Design review of the part built by this model. Coordinates are the model's own, in mm. A direction names the side the tool comes from. Round coordinates to 2 decimals unless told otherwise and drop trailing zeros. Loops run counter-clockwise (first coordinate to the right, second up) from the corner with the lowest first, then second, coordinate; pieces in that order, holes last. Notation, with made-up numbers: (87.5, 30) - (108.5, 30) arc R26 cw to (108.5, 54) - close; hole circle Ø7 at (-4.75, 58). An arc over 180 degrees is marked (long way). Return JSON: item names as keys, results as strings. Group by question number.
Autodesk Inventor part; units mm, degrees
ref_plane "Work Plane1" through (15, 0, 0) normal (0, 0, -1) x (-1, 0, 0)
ref_plane "YZ Plane" through (0, 0, 0) normal (1, 0, 0) x (0, 1, 0)
ref_plane "XZ Plane" through (0, 0, 0) normal (0, 1, 0) x (-1, 0, 0)
sketch "Sketch1" plane through (0, 0, 0) normal (0, 1, 0) x (-1, 0, 0)
  line L0 (-15, -17) -> (15, -17)
  line L1 (15, -17) -> (15, 17)
  line L2 (15, 17) -> (-15, 17)
  line L3 (-15, 17) -> (-15, -17)
  line L4 (-15, -17) -> (15, 17) construction
  line L5 (15, -17) -> (-15, 17) construction
  line L6 (-21, 0) -> (21, 0) construction
  line L7 (15, 10) -> (-15, 10) construction
  line L8 (11.85, 17) -> (11.85, -17) construction
  line L9 (0, -23.8) -> (0, 23.8) construction
  line L10 (-11.85, 17) -> (-11.85, -17) construction
  line L11 (15, -10) -> (-15, -10) construction
  circle A0 centre (11.85, 10) radius 1.5
  circle A1 centre (11.85, -10) radius 1.5
  circle A2 centre (-11.85, 0) radius 1.5
  point P0 (0, 0)
  dimension "d0" = 34
  dimension "d1" = 30
  dimension "d2" = 10
  dimension "d3" = 11.85
  dimension "d4" = 3
  dimension "d5" = 3
  dimension "d6" = 3
extrude "Extrusion1" add sketch "Sketch1" along normal blind 3.25
sketch "Sketch2" plane through (0, 3.25, 0) normal (0, 1, 0) x (1, 0, 0)
  line L0 (15, 17) -> (-15, 17)
  line L1 (15, -17) -> (15, 17)
  line L2 (-15, 17) -> (15, 17)
  line L3 (15, 17) -> (15, 15)
  line L4 (15, 15) -> (-15, 15)
  line L5 (-15, 15) -> (-15, 17)
  line L6 (21, 0) -> (-21, 0) construction
  line L7 (15, -17) -> (-15, -17)
  line L8 (15, 17) -> (15, -17)
  line L9 (15, -15) -> (-15, -15)
  line L10 (-15, -15) -> (-15, -17)
  point P0 (0, 0)
  dimension "d9" = 2
extrude "Extrusion2" add sketch "Sketch2" along normal blind 3
sketch "Sketch5" plane through (15, 0, -17) normal (0, 0, -1) x (-1, 0, 0)
  line L0 (0, 0) -> (30, 0)
  line L1 (30, 0) -> (30, 6.25)
  line L2 (0, 6.25) -> (30, 6.25)
  line L3 (0, 0) -> (0, 6.25)
  line L4 (0, 3.125) -> (4.65, 3.125) construction
  line L5 (4.65, 3.125) -> (19.35, 3.125) construction
  dimension "d40" = 4.65
  dimension "d41" = 14.7
sketch "Sketch8" plane through (0, 3.25, 0) normal (0, 1, 0) x (1, 0, 0)
  line L0 (15, 15) -> (-15, 15)
  line L1 (-15, 15) -> (-15, -15)
  line L2 (-15, -15) -> (15, -15)
  line L3 (15, -15) -> (15, 15)
  circle A0 centre (-11.85, -10) radius 1.5
  circle A1 centre (-11.85, 10) radius 1.5
  circle A2 centre (11.85, 0) radius 1.5
  line L4 (-9.35, -15) -> (-9.35, -8)
  line L5 (-9.35, -8) -> (0.65, -8)
  line L6 (0.65, -8) -> (0.65, -15)
  line L7 (15, -8) -> (5.35, -8)
  line L8 (5.35, -8) -> (5.35, -15)
  line L9 (15, -8) -> (15, -15)
  line L10 (15, -17) -> (15, 17)
  line L11 (15, -15) -> (5.35, -15)
  line L12 (0.65, -15) -> (-9.35, -15)
  line L13 (15, 0) -> (-15, 0) construction
  line L14 (-15, 17) -> (-15, -17) construction
  line L15 (-15, 15) -> (15, 15)
  line L16 (15, 15) -> (15, -15)
  line L17 (-9.35, 15) -> (-9.35, 8)
  line L18 (-9.35, 8) -> (0.65, 8)
  line L19 (0.65, 8) -> (0.65, 15)
  line L20 (15, 8) -> (5.35, 8)
  line L21 (5.35, 8) -> (5.35, 15)
  line L22 (15, 8) -> (15, 15)
  line L23 (15, 17) -> (15, -17)
  line L24 (15, 15) -> (5.35, 15)
  line L25 (0.65, 15) -> (-9.35, 15)
  circle A3 centre (11.85, 0) radius 4
  circle A4 centre (-11.85, 10) radius 4
  circle A5 centre (-11.85, -10) radius 4
  point P0 (0, 0)
  dimension "d34" = 9.65
  dimension "d35" = 4.7
  dimension "d36" = 10
  dimension "d37" = 8
  dimension "d44" = 8
extrude "Extrusion5" cut sketch "Sketch8" against normal through all contours L3 L20 L21 L0 | L19 L18 A4 L17 L0 | A4 L18 L17 | L3 L2 L8 L7 | A5 L4 L5 | L5 L6 L2 L4 A5
hole "Hole1" at (-4.35, 3.125, -17) at (10.35, 3.125, -17) direction (0, 0, 1) diameter 2.5 end up to surface
ref_plane "Work Plane1" through (15, 0, 0) normal (0, 0, -1) x (-1, 0, 0)
mirror "Mirror1" about plane through (15, 0, 0) normal (0, 0, -1) of "Hole1"
extrude "Extrusion6" add sketch "Sketch8" along normal blind 3 contours L21 L20 L3 A3 L7 L8 L2 L6 L5 A5 L1 A4 L18 L19 L0 | L3 A3 | L17 A4 L1 L0 | L17 L18 A4 L1 | A5 L5 L4 L1 | A5 L4 L2 L1 picked at (14.45, 0)
extrude "Extrusion7" cut sketch "Sketch8" along normal through all contours A3 L3 | L3 A3 | A4 L18 L17 | L17 L18 A4 L1 | L1 A4 | A5 L5 L4 L1 | L1 A5 | A5 L4 L5
fillet "Fillet3" radius 1.5 12 edges at (-9.35, 3.125, 15) (0.65, 3.125, -8) (-9.35, 1.625, -8) (5.35, 3.125, -8) (5.35, 3.125, 8) (-9.35, 1.625, 8) (0.65, 3.125, 8) (-9.35, 3.125, -15) (0.65, 3.125, -15) (5.35, 3.125, -15) (5.35, 3.125, 15) (0.65, 3.125, 15)
fillet "Fillet4" radius 1.5 2 edges at (15, 3.125, 8) (15, 3.125, -8)
equation "\"d0\" = fix_width"
equation "\"d1\" = fix_length"
equation "\"d7\" = first_layer_thickness"
equation "\"d10\" = thickness - first_layer_thickness"
equation "\"d40\" = side_fix_2_back"
equation "\"d41\" = side_fix_spacing"
equation "\"d34\" = side_fix_2_back + side_fix_clearance"
equation "\"d35\" = side_fix_spacing - 2 * side_fix_clearance"
equation "\"d36\" = 2 * side_fix_clearance"
equation "\"d37\" = cam_fix_clearance"
equation "\"d45\" = thickness - first_layer_thickness"
equation "\"d47\" = thickness - first_layer_thickness"
equation "\"fix_width\" = 34"
equation "\"side_fix_2_back\" = 4.65"
equation "\"side_fix_spacing\" = 14.7"
equation "\"side_fix_clearance\" = 5"
equation "\"cam_fix_clearance\" = 8"
equation "\"fix_length\" = 30"
equation "\"thickness\" = 6.25"
equation "\"first_layer_thickness\" = 3.25"
properties part number "ptgrey_fix2" material "Aluminum 6061"
Q1. Insertion check: pin 1 Ø3.5 at (x, z) = (-10.5, 9) entering from +Y; pin 2 Ø2.5 at (x, z) = (-11.85, -10) entering from +Y. Each pin has a flat end and moves straight along its axis. Give the tip position at first contact, or say it passes through.
Q2. Add section A-A, the plane x = -7. State the section outline as (y, z) points.
Q3. Add section D-D, the plane x = -11.85. State the section outline as (y, z) points, plus the area to 3 significant figures.
Q4. Add section C-C, the plane z = -10. State the section outline as (x, y) points.
Q5. Add section B-B, the plane z = 0. State the section outline as (x, y) points, plus the area to 3 significant figures.
Q6. For line 1 (Z direction, x = -6.25, y = 4.25); line 2 (Z direction, x = 11.85, y = 5.4); line 3 (Y direction, x = 10.35, z = 15.5) (3 decimals), list the stretches that pass through material, from the lowest coordinate up.
Q7. Draft analysis for pull direction X (two halves, no side actions). For faces 4 (the flat face through (10, 3, -8)), 5 (the cylindrical face through (5.8, 3.08, -8.43)), 6 (the flat face through (-4, 5, 15)), state which applies: pulls with the +X half, pulls with the -X half, needs draft (parallel to the pull), parting line crosses it, or undercut.
Q8. Tool access review of faces 1 (the flat face through (12, 3, -15)), 2 (the flat face through (11, 3.25, 2)), 3 (the cylindrical face through (-8.72, 2.39, 8.28)): name each direction out of +Z, -Z, +X, -X, +Y, -Y from which nothing blocks a thin tool from reaching the whole face with its end or side.
Evaluation:
{
 "1": {"pin 1": "y = 3.25", "pin 2": "through"},
 "2": {"outline": "(0, -17) - (6.25, -17) - (6.25, -15) - (0, -15) - close; (0, -8) - (6.25, -8) - (6.25, 8) - (0, 8) - close; (0, 15) - (6.25, 15) - (6.25, 17) - (0, 17) - close"},
 "3": {"outline": "(0, -17) - (6.25, -17) - (6.25, -14) - (3.25, -14) - (3.25, -11.5) - (0, -11.5) - close; (0, -8.5) - (3.25, -8.5) - (3.25, -6) - (6.25, -6) - (6.25, 6) - (3.25, 6) - (3.25, 8.5) - (0, 8.5) - close; (0, 11.5) - (3.25, 11.5) - (3.25, 14) - (6.25, 14) - (6.25, 17) - (0, 17) - close", "area": "145 mm²"},
 "4": {"outline": "(-15, 0) - (-13.35, 0) - (-13.35, 3.25) - (-15, 3.25) - close; (-10.35, 0) - (-9.35, 0) - (-9.35, 3.25) - (-10.35, 3.25) - close; (0.65, 0) - (5.35, 0) - (5.35, 6.25) - (0.65, 6.25) - close"},
 "5": {"outline": "(-15, 0) - (10.35, 0) - (10.35, 3.25) - (7.85, 3.25) - (7.85, 6.25) - (-15, 6.25) - close; (13.35, 0) - (15, 0) - (15, 3.25) - (13.35, 3.25) - close", "area": "156 mm²"},
 "6": {"line 1": "-17 to -15, -8 to 8, 15 to 17", "line 2": "-17 to -15, -8 to -4, 4 to 8, 15 to 17", "line 3": "0 to 1.875, 4.375 to 6.25"},
 "7": {"face 4": "needs draft", "face 5": "pulls with the +X half", "face 6": "undercut"},
 "8": {"face 1": "+X, +Y, -Y", "face 2": "+Y", "face 3": "+Y, -Y"}
}
